Read the model definition and answer for the solid it produces. Units are mm, in the model's axes. A direction names the side the tool comes from. Coordinates: 2 decimals unless noted, no trailing zeros. Write each loop counter-clockwise with the first axis right and the second up, starting at its lowest first coordinate (ties: lowest second). Pieces come first, ordered by that corner, then holes. Notation, with made-up numbers: (71, -32) - (78, -32) arc R29 ccw to (78, 4) - close; hole circle Ø1 at (-9, -8). An arc over 180 degrees is marked (long way). Use a Markdown table: item, result.
from build123d import *

# Parameters (mm, degrees)
SKIZZE1_W                       = 120
SKIZZE1_H                       = 120
LINEAR_AUSTRAGEN1_DEPTH         = 10
VERRUNDUNG2_R                   = 10
VERRUNDUNG2_OF_SPIEGELN1_R      = 10
SKIZZE3_W                       = 170
SKIZZE3_H                       = 60
SCHNITT_LINEAR_AUSTRAGEN1_DEPTH = 10
VERRUNDUNG3_R                   = 3
SCHNITT_LINEAR_AUSTRAGEN2_DEPTH = 10
SKIZZE5_W                       = 14
SKIZZE5_H                       = 2
SCHNITT_LINEAR_AUSTRAGEN3_DEPTH = 2


with BuildPart() as part:
    # Skizze1 → Linear austragen1 (new body)
    with BuildSketch(Plane(origin=(0, 10, 0), x_dir=(1, 0, 0), z_dir=(0, 1, 0))):
        with BuildLine():
            Line((0, -75), (130, -75))
            ThreePointArc((130, -75), (144.142135624, -69.142135624), (150, -55))
            Line((150, -55), (150, 75))
            Line((150, 75), (150, 150))
            Line((150, 150), (0, 150))
            Line((0, 150), (0, 75))
            Line((0, 75), (0, -75))
        make_face()
        with Locations((75, 0)):
            Rectangle(SKIZZE1_W, SKIZZE1_H, mode=Mode.SUBTRACT)
    linear_austragen1 = extrude(amount=LINEAR_AUSTRAGEN1_DEPTH)

    # Verrundung2
    verrundung2_edges = [part.edges().sort_by_distance(p)[0] for p in [
        (15, 15, -60),
        (15, 15, 60),
        (135, 15, 60),
        (135, 15, -60),
    ]]
    fillet(verrundung2_edges, radius=VERRUNDUNG2_R)

    # Spiegeln1: Linear austragen1 across plane
    add(linear_austragen1.mirror(Plane(origin=(0, 20, -150), x_dir=(0, 0, 1), z_dir=(1, 0, 0))))

    # Verrundung2 of Spiegeln1
    verrundung2_of_spiegeln1_edges = [part.edges().sort_by_distance(p)[0] for p in [
        (-15, 15, -60),
        (-15, 15, 60),
        (-135, 15, 60),
        (-135, 15, -60),
    ]]
    fillet(verrundung2_of_spiegeln1_edges, radius=VERRUNDUNG2_OF_SPIEGELN1_R)

    # Skizze3 → Schnitt-Linear austragen1 (cut)
    with BuildSketch(Plane.XZ.offset(-10)):
        with Locations((-35, -110)):
            Rectangle(SKIZZE3_W, SKIZZE3_H)
    extrude(amount=-SCHNITT_LINEAR_AUSTRAGEN1_DEPTH, mode=Mode.SUBTRACT)

    # Verrundung3
    verrundung3_edges = [part.edges().sort_by_distance(p)[0] for p in [
        (-120, 15, -140),
        (-120, 15, -80),
        (50, 15, -80),
        (50, 15, -140),
    ]]
    fillet(verrundung3_edges, radius=VERRUNDUNG3_R)

    # Skizze4 → Schnitt-Linear austragen2 (cut)
    with BuildSketch(Plane.XZ.offset(-10)):
        with BuildLine():
            Line((-3.000050853, 75), (-3.000050853, 68))
            ThreePointArc((-3.000050853, 68), (0.008683003, 65.000012713), (2.999898294, 68.017467638))
            Line((2.999898294, 68.017467638), (2.959241489, 75))
            Line((2.959241489, 75), (-3.000050853, 75))
        make_face()
    extrude(amount=-SCHNITT_LINEAR_AUSTRAGEN2_DEPTH, mode=Mode.SUBTRACT)

    # Skizze5 → Schnitt-Linear austragen3 (cut)
    with BuildSketch(Plane.XZ.offset(-10)):
        with Locations((-0.020404682, 71)):
            Rectangle(SKIZZE5_W, SKIZZE5_H)
    extrude(amount=-SCHNITT_LINEAR_AUSTRAGEN3_DEPTH, mode=Mode.SUBTRACT)


solid = part.part
(1) A cutting plane is placed at D-D, the plane x = 76.5. Write down the section's boundary in (y, z).
Report:
| item | result |
|---|---|
| outline | (10, -150) - (20, -150) - (20, -60) - (10, -60) - close; (10, 60) - (20, 60) - (20, 75) - (10, 75) - close |
(2) Each of these flat-tipped pins is pushed along its axis until it touches: P1, Ø1, axis at y = 10.5, z = 71.5, coming from the -X side; P2, Ø1.5, axis at x = -108, z = -59.5, coming from the -Y side; P3, Ø2, axis at y = 11, z = 71.5, coming from the +X side. Where does it stop, or does it pass through?
Report:
| item | result |
|---|---|
| P1 | stops at x = -142 |
| P2 | stops at y = 10 |
| P3 | stops at x = 142.64 |
(3) The mould has two halves that part along Z. Classify faces 4 (the flat face through (-150, 15, -46)), 5 (the flat face through (-2, 15, -150)), 6 (the cylindrical face through (143.986, 14.93, 69.297)), 7 (the flat face through (50, 15, -110)): pulls with the +Z half, pulls with the -Z half, needs draft (parallel to the pull), parting line crosses it, or undercut.
Report:
| item | result |
|---|---|
| face 4 | needs draft |
| face 5 | pulls with the -Z half |
| face 6 | pulls with the +Z half |
| face 7 | undercut |
(4) For faces 1 (the flat face through (-3, 15, 72)), 2 (the flat face through (-66, 15, 75)), 3 (the flat face through (15, 15, 1)), determine the directions among +Z, -Z, +X, -X, +Y, -Y from which every point of the face is accessible in a straight line to the end or side of a thin tool.
Report:
| item | result |
|---|---|
| face 1 | +Z, +Y, -Y |
| face 2 | +Z, +X, -X, +Y, -Y |
| face 3 | +Y, -Y |
(5) Straight lines are drawn through the part: L1, parallel to X at y = 11.25, z = -40; L2, parallel to Z at x = -99.5, y = 11.5; L3, parallel to X at y = 13.75, z = -128. For each, find the intervals that lie inside material, in ascending order.
Report:
| item | result |
|---|---|
| L1 | x = -150 to -135, -15 to 15, 135 to 150 |
| L2 | z = -150 to -140, -80 to -60, 60 to 75 |
| L3 | x = -150 to -120, 50 to 150 |
(6) A cutting plane is placed at B-B, the plane y = 18. Count the separate pieces of the cut face and the enclosed holes in it, and give its area (3 significant figures).
Report:
| item | result |
|---|---|
| separate pieces | 1 |
| enclosed holes | 3 |
| area | 28,500 mm² |
(7) A cutting plane is placed at C-C, the plane x = -78. Write down the section's boundary in (y, z), and give its area (3 significant figures).
Report:
| item | result |
|---|---|
| outline | (10, -150) - (20, -150) - (20, -140) - (10, -140) - close; (10, -80) - (20, -80) - (20, -60) - (10, -60) - close; (10, 60) - (20, 60) - (20, 75) - (10, 75) - close |
| area | 450 mm² |
(8) A cutting plane is placed at A-A, the plane z = -41. Write down the section's boundary in (x, y), and give its area (3 significant figures).
Report:
| item | result |
|---|---|
| outline | (-150, 10) - (-135, 10) - (-135, 20) - (-150, 20) - close; (-15, 10) - (15, 10) - (15, 20) - (-15, 20) - close; (135, 10) - (150, 10) - (150, 20) - (135, 20) - close |
| area | 600 mm² |
